Part model, mm, in its own coordinate system. Face numbers are marked on the shaded views. A direction names the side the tool comes from. Round coordinates to 2 decimals unless told otherwise and drop trailing zeros. Order: outer loops, then holes, each group sorted by start corner. A loop starts at its lowest first (then second) coordinate and runs counter-clockwise, first axis right, second up. Notation, with made-up numbers: M -2,-32 L 15,-32 A15 cw 15,-20 Z; hole C 18.25,46.5 d5. An arc over 180 degrees is marked long. Write each question's results on one line, items separated by ' | '. Start each with the question number.
1. Two-plate mould, pull along X, no slides. Class the marked faces 1, 2 and 3: +X half, -X half, draft (parallel to the pull), parting line (faces both ways), or undercut.
2. Drop flat-ended pins along their axis: pin 1 Ø1.1 at (y, z) = (34.5, 4.5) entering from -X; pin 2 Ø1.5 at (x, z) = (-1, 6) entering from -Y; pin 3 Ø0.5 at (y, z) = (34.5, 4) entering from +X. Give the stop position or say it passes through.
3. Probe L1, parallel to X at y = 6, z = 7.75; L2, parallel to Y at x = -1, z = 4.25; L3, parallel to X at y = 7, z = 1.75. List the from-to ranges inside material, lowest first. Write a range as [from, to].
4. Band-saw the part on D-D, the plane y = 3. List the corners of the cut face in (x, z), then the cut area to 3 significant figures.
5. Band-saw the part on B-B, the plane y = 15. List the corners of the cut face in (x, z), then the cut area to 3 significant figures.
6. Band-saw the part on C-C, the plane z = 6. List the corners of the cut face in (x, y) (1 decimal).
7. Band-saw the part on A-A, the plane x = 0. List the corners of the cut face in (y, z).
8. Which spindle directions (+Z, -Z, +X, -X, +Y, -Y) get a long thin tool onto all of the face, cutting with end or side? Do the marked faces 4 and 5. Say none if no direction does.
```python
from build123d import *

# Parameters (mm, degrees)
ESQUISSE1_R        = 2
BOSS_EXTRU_2_DEPTH = 9


with BuildPart() as part:
    # Esquisse1 → Boss.-Extru.2 (new body)
    with BuildSketch(Plane.XY):
        with BuildLine():
            Line((6.5, 35), (-6.5, 35))
            Line((-6.5, 35), (-6.5, 34))
            Line((-6.5, 34), (-8.5, 34))
            Line((-8.5, 34), (-13.5, 29))
            Line((-13.5, 29), (-13.5, 10))
            ThreePointArc((-13.5, 10), (0, 0), (13.5, 10))
            Line((13.5, 10), (13.5, 29))
            Line((13.5, 29), (8.5, 34))
            Line((8.5, 34), (6.5, 34))
            Line((6.5, 34), (6.5, 35))
        make_face()
        with Locations((0, 15)):
            Circle(ESQUISSE1_R, mode=Mode.SUBTRACT)
    extrude(amount=BOSS_EXTRU_2_DEPTH)


solid = part.part
```
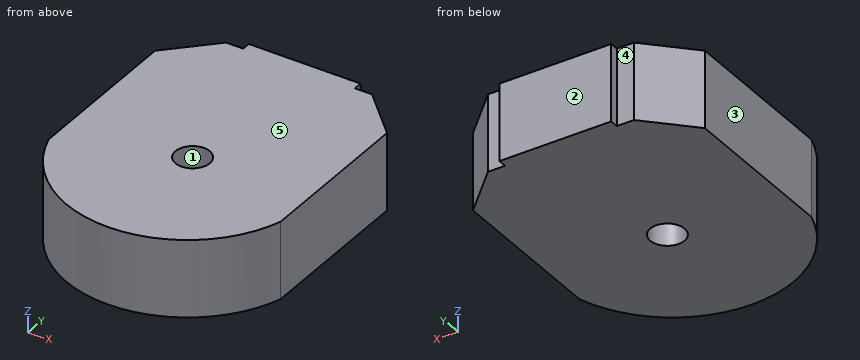
Solution:
1) face 1: undercut | face 2: draft | face 3: -X half
2) pin 1: x = -8.55 | pin 2: y = 0 | pin 3: x = 6.5
3) L1: [-11.55, 11.55] | L2: [0.04, 13.27], [16.73, 35] | L3: [-12.19, 12.19]
4) outline: M -8.7,0 L 8.7,0 L 8.7,9 L -8.7,9 Z | area: 157 mm^2
5) outline: M -13.5,0 L -2,0 L -2,9 L -13.5,9 Z; M 2,0 L 13.5,0 L 13.5,9 L 2,9 Z | area: 207 mm^2
6) outline: M -13.5,10 A14.1 ccw 13.5,10 L 13.5,29 L 8.5,34 L 6.5,34 L 6.5,35 L -6.5,35 L -6.5,34 L -8.5,34 L -13.5,29 Z; hole C 0,15 d4
7) outline: M 0,0 L 13,0 L 13,9 L 0,9 Z; M 17,0 L 35,0 L 35,9 L 17,9 Z
8) face 4: +Z, -Z, -X, +Y | face 5: +Z, +X, -X, +Y, -Y
